Design review of the part built by this model. Coordinates are the model's own, in mm. Face numbers are marked on the shaded views. Round coordinates to 2 decimals unless told otherwise and drop trailing zeros. Loops run counter-clockwise (first coordinate to the right, second up) from the corner with the lowest first, then second, coordinate; pieces in that order, holes last. Notation, with made-up numbers: (-16, -18) -> (42, -18) arc R29 cw to (42, 2) -> close; hole circle Ø4 at (33, 32.5). An arc over 180 degrees is marked (long way). Answer as CSV lines item,"result". Start each with the question number.
(1) Take a section at D-D, the plane z = 20. Write out the cut boundary in (x, y), and give its area (3 significant figures).
(2) Take a section at A-A, the plane x = -19.5. Write out the cut boundary in (y, z), and give its area (3 significant figures).
(3) For P1, Ø5, axis at x = -188, y = -76.5, coming from the +Z side; P2, Ø8, axis at y = 35.5, z = 48.5, coming from the -X side, all flat-tipped, find the tip position at first contact; note any pin that passes through.
(4) Draft analysis for pull direction Y (two halves, no side actions). For the marked faces 1, 2 and 3, state which applies: +Y half, -Y half, draft (parallel to the pull), parting line (faces both ways), or undercut.
(5) To check wall thickness, follow line 1 (Y direction, x = 188, z = 1.7); line 2 (X direction, y = 60, z = 45.5); line 3 (Y direction, x = 3.5, z = 10.5). State the ranges of each line that lie inside material, in increasing order. Write a range as from..to.
(6) Take a section at C-C, the plane z = 58.5. Write out the cut boundary in (x, y).
(7) Take a section at B-B, the plane y = 18.5. Write out the cut boundary in (x, z), and give its area (3 significant figures).
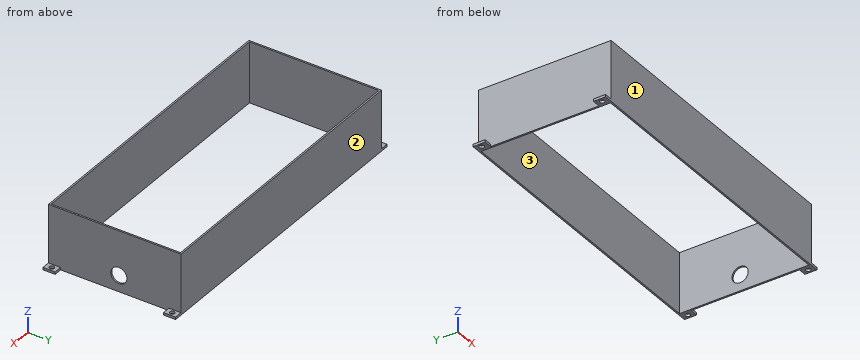
from build123d import *

# Parameters (mm, degrees)
SKETCH_1_W          = 366
SKETCH_1_H          = 164
SKETCH_1_W_2        = 362
SKETCH_1_H_2        = 160
EXTRUDE_1_DEPTH     = 75
SKETCH_2_W          = 3
SKETCH_2_H          = 15
EXTRUDE_2_DEPTH     = 10
SKETCH_3_R          = 3
CUT_EXTRUDE_1_DEPTH = 10
SKETCH_4_R          = 10
CUT_EXTRUDE_2_DEPTH = 10


with BuildPart() as part:
    # 草圖1 → 填料-伸長1 (new body)
    with BuildSketch(Plane.XY):
        Rectangle(SKETCH_1_W, SKETCH_1_H)
        Rectangle(SKETCH_1_W_2, SKETCH_1_H_2, mode=Mode.SUBTRACT)
    extrude(amount=EXTRUDE_1_DEPTH)

    # 草圖2 → 填料-伸長2 (add)
    with BuildSketch(Plane(origin=(183, 0, 0), x_dir=(0, 0, -1), z_dir=(1, 0, 0))):
        with Locations((-1.5, 74.5)):
            Rectangle(SKETCH_2_W, SKETCH_2_H)
        with Locations((-1.5, -74.5)):
            Rectangle(SKETCH_2_W, SKETCH_2_H)
    extrude_2 = extrude(amount=EXTRUDE_2_DEPTH)

    # 鏡射1: 填料-伸長2 across plane
    add(extrude_2.mirror(Plane(origin=(0, 0, 0), x_dir=(0, 0, 1), z_dir=(1, 0, 0))))

    # 草圖3 → 除料-伸長1 (cut)
    with BuildSketch(Plane.XY.offset(3)):
        with Locations((188, 74.5)):
            Circle(SKETCH_3_R)
        with Locations((188, -74.5)):
            Circle(SKETCH_3_R)
    cut_extrude_1 = extrude(amount=-CUT_EXTRUDE_1_DEPTH, mode=Mode.SUBTRACT)

    # 鏡射3: 除料-伸長1 across plane
    add(cut_extrude_1.mirror(Plane(origin=(0, 0, 0), x_dir=(0, 0, 1), z_dir=(1, 0, 0))), mode=Mode.SUBTRACT)

    # 草圖4 → 除料-伸長2 (cut)
    with BuildSketch(Plane(origin=(183, 0, 0), x_dir=(0, 0, -1), z_dir=(1, 0, 0))):
        with Locations(Location((-20, 5, 0), (0, 0, 90))):
            Circle(SKETCH_4_R)
    extrude(amount=-CUT_EXTRUDE_2_DEPTH, mode=Mode.SUBTRACT)


solid = part.part
The answers:
1,outline,"(-183, -82) -> (183, -82) -> (183, -5) -> (181, -5) -> (181, -80) -> (-181, -80) -> (-181, 80) -> (181, 80) -> (181, 15) -> (183, 15) -> (183, 82) -> (-183, 82) -> close"
1,area,"2,060 mm²"
2,outline,"(-82, 0) -> (-80, 0) -> (-80, 75) -> (-82, 75) -> close; (80, 0) -> (82, 0) -> (82, 75) -> (80, 75) -> close"
2,area,"300 mm²"
3,P1,"z = 3"
3,P2,"x = -183"
4,face 1,"-Y half"
4,face 2,"+Y half"
4,face 3,"undercut"
5,line 1,"-82..-77.5, -71.5..-67, 67..71.5, 77.5..82"
5,line 2,"-183..-181, 181..183"
5,line 3,"-82..-80, 80..82"
6,outline,"(-183, -82) -> (183, -82) -> (183, 82) -> (-183, 82) -> close; hole (-181, -80) -> (181, -80) -> (181, 80) -> (-181, 80) -> close"
7,outline,"(-183, 0) -> (-181, 0) -> (-181, 75) -> (-183, 75) -> close; (181, 0) -> (183, 0) -> (183, 75) -> (181, 75) -> close"
7,area,"300 mm²"
